Read the model definition and answer for the solid it produces. Units are mm, in the model's axes. A direction names the side the tool comes from. Coordinates: 2 decimals unless noted, no trailing zeros. Write each loop counter-clockwise with the first axis right and the second up, starting at its lowest first coordinate (ties: lowest second). Pieces come first, ordered by that corner, then holes.
1) Find the intervals of material crossed by line 1 (Z direction, x = 11, y = -2.5); line 2 (X direction, y = 5.5, z = 1.5); line 3 (X direction, y = 5.5, z = 9.75), in increasing order.
2) The part is cut by section B-B (x = 13). Determine the outline of the cut face in (y, z).
3) The part is cut by section D-D (y = -3.25). Determine the outline of the cut face in (x, z).
4) Which of the six approach directions +Z, -Z, +X, -X, +Y, -Y give full straight-line access (tool end or side, diameter ignored) to faces 1 (the face through (-13.592, 0, 9)), 2 (the face through (-14.5, 4, 5)), 3 (the face through (-16, -5, 4)), 4 (the face through (18, 0, 8))?
5) Determine the mould class of faces 5 (the face through (0, 0, 6.537)), 6 (the face through (-16, 5, 4)), 7 (the face through (14, 0, 10)) for opening direction X: +X half, -X half, draft (parallel to the pull), parting line (faces both ways), or undercut.
6) The part is cut by section C-C (z = 1.25). Determine the outline of the cut face in (x, y).
7) The part is cut by section A-A (z = 4.25). Determine the outline of the cut face in (x, y), then the cut area to 3 significant figures.
8) Each of these flat-tipped pins is pushed along its axis until it touches: pin 1 Ø1 at (y, z) = (4.5, 3.5) entering from +X; pin 2 Ø4.5 at (x, y) = (-12, -1.5) entering from +Z; pin 3 Ø3 at (y, z) = (2.5, 0.5) entering from -X; pin 4 Ø6 at (x, y) = (-4.5, 1.5) entering from -Z. Where does it stop, or does it pass through?
from build123d import *

# Parameters (mm, degrees)
F0_W     = 32
F0_H     = 15
F1_DEPTH = 8
F2_W     = 29
F2_H     = 3.8
F3_DEPTH = 30
F5_DEPTH = 2
F6_W     = 20.6003077328
F6_H     = 15
F7_DEPTH = 5
F8_DEPTH = 25


with BuildPart() as f1:
    # F0 (on Top) → F1 (new body)
    with BuildSketch(Plane.XY):
        Rectangle(F0_W, F0_H)
    extrude(amount=F1_DEPTH)

    # F2 (on face) → F3 (cut)
    with BuildSketch(Plane.XZ.offset(7.5)):
        with Locations((0, 4.6374863014)):
            Rectangle(F2_W, F2_H)
    extrude(amount=-F3_DEPTH, mode=Mode.SUBTRACT)

    # F4 (on face) → F5 (join)
    with BuildSketch(Plane.XY.offset(8)):
        with BuildLine():
            Line((18.3776282892, 7.5), (16, 7.5))
            Line((16, 7.5), (16, 1.6))
            ThreePointArc((16, 1.6), (17.1313708499, 1.1313708499), (17.6, 0))
            ThreePointArc((17.6, 0), (17.1313708499, -1.1313708499), (16, -1.6))
            Line((16, -1.6), (16, -7.5))
            Line((16, -7.5), (18.3776282892, -7.5))
            Line((18.3776282892, -7.5), (18.3776282892, 7.5))
        make_face()
        with BuildLine():
            Line((16, 7.5), (13.3776282892, 7.5))
            Line((13.3776282892, 7.5), (13.3776282892, -7.5))
            Line((13.3776282892, -7.5), (16, -7.5))
            Line((16, -7.5), (16, -1.6))
            ThreePointArc((16, -1.6), (14.4, 0), (16, 1.6))
            Line((16, 1.6), (16, 7.5))
        make_face()
        with BuildLine():
            Line((-16, 1.6), (-16, 7.5))
            Line((-16, 7.5), (-18.5922654346, 7.5))
            Line((-18.5922654346, 7.5), (-18.5922654346, -7.5))
            Line((-18.5922654346, -7.5), (-16, -7.5))
            Line((-16, -7.5), (-16, -1.6))
            ThreePointArc((-16, -1.6), (-17.6, 0), (-16, 1.6))
        make_face()
        with BuildLine():
            Line((-13.5922654346, -7.5), (-13.5922654346, 7.5))
            Line((-13.5922654346, 7.5), (-16, 7.5))
            Line((-16, 7.5), (-16, 1.6))
            ThreePointArc((-16, 1.6), (-14.8686291501, 1.1313708499), (-14.4, 0))
            ThreePointArc((-14.4, 0), (-14.8686291501, -1.1313708499), (-16, -1.6))
            Line((-16, -1.6), (-16, -7.5))
            Line((-16, -7.5), (-13.5922654346, -7.5))
        make_face()
    extrude(amount=F5_DEPTH)

    # F6 (on face) → F7 (cut)
    with BuildSketch(Plane(origin=(0, 0, 0), x_dir=(1, 0, 0), z_dir=(0, 0, -1))):
        Rectangle(F6_W, F6_H)
    extrude(amount=-F7_DEPTH, mode=Mode.SUBTRACT)

    # F4 (on face) → F8 (cut)
    with BuildSketch(Plane.XY.offset(8)):
        with BuildLine():
            ThreePointArc((-14.4, 0), (-14.8686291501, 1.1313708499), (-16, 1.6))
            Line((-16, 1.6), (-16, -1.6))
            ThreePointArc((-16, -1.6), (-14.8686291501, -1.1313708499), (-14.4, 0))
        make_face()
        with BuildLine():
            Line((-16, -1.6), (-16, 1.6))
            ThreePointArc((-16, 1.6), (-17.6, 0), (-16, -1.6))
        make_face()
        with BuildLine():
            Line((16, -1.6), (16, 1.6))
            ThreePointArc((16, 1.6), (14.4, 0), (16, -1.6))
        make_face()
        with BuildLine():
            ThreePointArc((17.6, 0), (17.1313708499, 1.1313708499), (16, 1.6))
            Line((16, 1.6), (16, -1.6))
            ThreePointArc((16, -1.6), (17.1313708499, -1.1313708499), (17.6, 0))
        make_face()
    extrude(amount=-F8_DEPTH, mode=Mode.SUBTRACT)


solid = f1.part
Reported:
1. line 1: z = 0 to 2.74, 6.54 to 8
1. line 2: x = -16 to -10.3, 10.3 to 16
1. line 3: x = -18.59 to -13.59, 13.38 to 18.38
2. outline: (-7.5, 0) - (7.5, 0) - (7.5, 2.74) - (-7.5, 2.74) - close; (-7.5, 6.54) - (7.5, 6.54) - (7.5, 8) - (-7.5, 8) - close
3. outline: (-18.59, 8) - (-16, 8) - (-16, 0) - (-10.3, 0) - (-10.3, 2.74) - (-14.5, 2.74) - (-14.5, 6.54) - (14.5, 6.54) - (14.5, 2.74) - (10.3, 2.74) - (10.3, 0) - (16, 0) - (16, 8) - (18.38, 8) - (18.38, 10) - (13.38, 10) - (13.38, 8) - (-13.59, 8) - (-13.59, 10) - (-18.59, 10) - close
4. face 1: +Z, +Y, -Y
4. face 2: +Y, -Y
4. face 3: -Z, -X, +Y, -Y
4. face 4: -Z, +X, +Y, -Y
5. face 5: undercut
5. face 6: -X half
5. face 7: draft
6. outline: (-16, -7.5) - (-10.3, -7.5) - (-10.3, 7.5) - (-16, 7.5) - (-16, 1.6) arc R1.6 cw to (-16, -1.6) - close; (10.3, -7.5) - (16, -7.5) - (16, -1.6) arc R1.6 cw to (16, 1.6) - (16, 7.5) - (10.3, 7.5) - close
7. outline: (-16, -7.5) - (-14.5, -7.5) - (-14.5, -0.56) arc R1.6 cw to (-16, -1.6) - close; (-16, 1.6) arc R1.6 cw to (-14.5, 0.56) - (-14.5, 7.5) - (-16, 7.5) - close; (14.5, -7.5) - (16, -7.5) - (16, -1.6) arc R1.6 cw to (14.5, -0.56) - close; (14.5, 0.56) arc R1.6 cw to (16, 1.6) - (16, 7.5) - (14.5, 7.5) - close
7. area: 37.1 mm2
8. pin 1: stops at x = 16
8. pin 2: stops at z = 10
8. pin 3: stops at x = -16
8. pin 4: stops at z = 6.54
